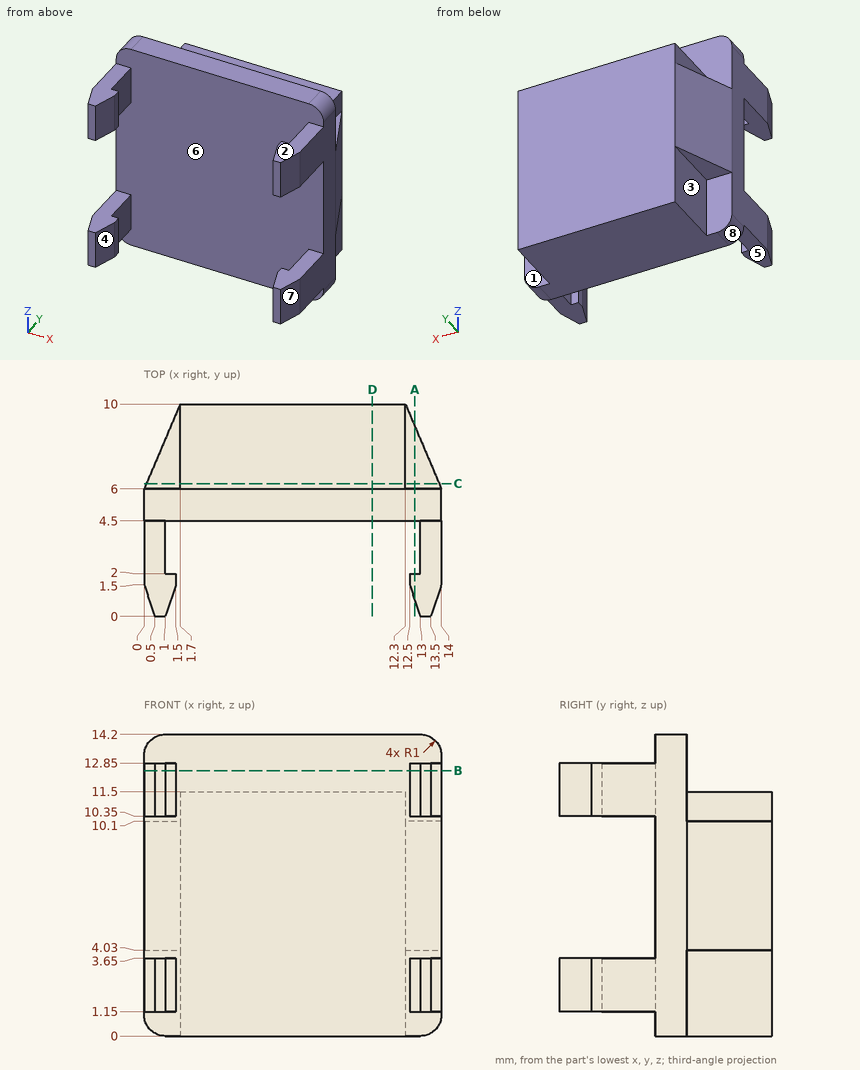
Input: dimensioned drawing with shaded views. Units: mm. Origin: part minimum x, y, z. A direction names the side the tool comes from. Give positions to 0.01 mm unless a question says otherwise; leave off trailing zeros. Write each loop counter-clockwise with the first axis right and the second up, starting at its lowest first coordinate (ties: lowest second). Pieces come first, ordered by that corner, then holes. Notation, with made-up numbers: M -3,-5.75 L 32,-5.75 A22 ccw 32,23.25 Z; hole C -28,-33 d6. An arc over 180 degrees is marked long. Write item = value, one per line. Start each with the question number.
1) Reachability of the marked faces 1, 2, 3, 4 and 5 from +Z, -Z, +X, -X, +Y, -Y: full face, straight path, thin tool, end or side. Return the list, or none.
2) Cut plane B-B on z = 12.5. Return the cut outline in (x, y).
3) Cut plane A-A on x = 12.75. Return the cut outline in (y, z), then the cut area to 3 significant figures.
4) First-contact query: pin 1 Ø4 at (y, z) = (9, 4) entering from +X; pin 2 Ø4 at (x, z) = (4.5, 3.5) entering from -Y; pin 3 Ø1.1 at (y, z) = (8.5, 11) entering from -X; pin 4 Ø6 at (x, y) = (7, 3) entering from -Z. Flat tips, straight axial feed; report the tip coordinate or a pass-through.
5) Material intervals for line 1 along Y through (x, z) = (4.5, 7); line 2 along Z through (x, y) = (5.5, 7.75); line 3 along X through (y, z) = (6.25, 10.75), sorted ascending. Write a range as [from, to].
6) Cut plane D-D on x = 10.75. Return the cut outline in (y, z).
7) Cut plane C-C on y = 6.25. Return the cut outline in (x, z), then the cut area to 3 significant figures.
8) Draft query along X for the marked faces 6, 7 and 8. Return one class per face: +X half, -X half, draft (parallel to the pull), parting line (faces both ways), or undercut.
Solved:
q1.face_1 = -Z, +X, +Y
q1.face_2 = +Z, +X, -X, -Y
q1.face_3 = -Z, -X, +Y
q1.face_4 = +Z, -Z, -Y
q1.face_5 = -Z, +X, -X, -Y
q2.outline = M 0,1.5 L 0.5,0 L 1,0 L 1.5,1.5 L 1.5,2 L 1,2 L 1,4.5 L 13,4.5 L 13,2 L 12.5,2 L 12.5,1.5 L 13,0 L 13.5,0 L 14,1.5 L 14,6 L 0,6 Z
q3.outline = M 0.75,1.15 L 2,1.15 L 2,3.65 L 0.75,3.65 Z; M 0.75,10.35 L 2,10.35 L 2,12.85 L 0.75,12.85 Z; M 4.5,0 L 6,0 L 6,4.03 L 8.94,4.03 L 8.94,10.1 L 6,10.1 L 6,14.2 L 4.5,14.2 Z
q3.area = 45.4 mm2
q4.pin_1 = 13.57
q4.pin_2 = 4.5
q4.pin_3 = 1.7
q4.pin_4 = 0
q5.line_1 = [4.5, 10]
q5.line_2 = [0, 11.5]
q5.line_3 = [1.7, 12.3]
q6.outline = M 4.5,0 L 10,0 L 10,11.5 L 6,11.5 L 6,14.2 L 4.5,14.2 Z
q7.outline = M 0.11,4.03 L 1.7,4.03 L 1.7,0 L 12.3,0 L 12.3,4.03 L 13.89,4.03 L 13.89,10.1 L 12.3,10.1 L 12.3,11.5 L 1.7,11.5 L 1.7,10.1 L 0.11,10.1 Z
q7.area = 141 mm2
q8.face_6 = undercut
q8.face_7 = +X half
q8.face_8 = -X half
